```python
from build123d import *

# Parameters (mm, degrees)
SKETCH1_R      = 2
EXTRUDE1_DEPTH = 12
CHAMFER1_SIZE  = 0.25
CHAMFER2_SIZE  = 0.5
EXTRUDE2_DEPTH = 1.5


with BuildPart() as part:
    # Sketch1 → Extrude1 (new body)
    with BuildSketch(Plane(origin=(0, 0, 0), x_dir=(1, 0, 0), z_dir=(0, 1, 0))):
        with Locations(Location((0, 0, 0), (0, 0, 270))):
            Circle(SKETCH1_R)
    extrude(amount=EXTRUDE1_DEPTH)

    # Chamfer1
    chamfer1_edges = [part.edges().sort_by_distance(p)[0] for p in [
        (0, 12, -2),
    ]]
    chamfer(chamfer1_edges, length=CHAMFER1_SIZE)

    # Chamfer2
    chamfer2_edges = [part.edges().sort_by_distance(p)[0] for p in [
        (0, 0, -2),
    ]]
    chamfer(chamfer2_edges, length=CHAMFER2_SIZE)

    # Sketch2 → Extrude2 (cut)
    with BuildSketch(Plane(origin=(0, 12, 0), x_dir=(1, 0, 0), z_dir=(0, 1, 0))):
        Polygon((-1.154700538, 0), (-0.577350269, -1), (0.577350269, -1), (1.154700538, 0), (0.577350269, 1), (-0.577350269, 1), align=None)
    extrude(amount=-EXTRUDE2_DEPTH, mode=Mode.SUBTRACT)


solid = part.part
```
The model under review builds one solid part; all positions refer to its coordinate system, in mm. A direction names the side the tool comes from. Round coordinates to 2 decimals unless told otherwise and drop trailing zeros. Loops run counter-clockwise (first coordinate to the right, second up) from the corner with the lowest first, then second, coordinate; pieces in that order, holes last. Notation, with made-up numbers: (82.25, -24.5) - (123.25, -24.5) arc R8 ccw to (123.25, -18.5) - close; hole circle Ø1 at (53.5, 32). An arc over 180 degrees is marked (long way). Use a Markdown table: item, result. Add a question column.
Q1. For probe 1 along Y at (x, z) = (0.8, -0.35); probe 2 along Z at (x, y) = (-1.5, 1.5); probe 3 along X at (y, z) = (7, -1.7), list the stretches that pass through material, from the lowest coordinate up.
Q2. Insertion check: pin 1 Ø1.5 at (y, z) = (8.5, -1) entering from -X. The pin has a flat end and moves straight along its axis. Give the tip position at first contact, or say it passes through.
Q3. The part is to be moulded in two halves that separate along Z. For faces 3 (the face through (-2, 6, 0)), 4 (the face through (0, 10.5, 0)), 5 (the face through (0, 0, 0)), say which applies: pulls with the +Z half, pulls with the -Z half, needs draft (parallel to the pull), parting line crosses it, or undercut.
Q4. Machinability: for faces 1 (the face through (0.86, 11.26, 0.51)), 2 (the face through (-1, 12, 1)), which of the approach directions +Z, -Z, +X, -X, +Y, -Y give a long, thin tool a straight path to every point of the face, cutting with its end or side? Answer none if there is none.
Q5. Add section A-A (y = 11.25). State the section outline as (x, z) points.
Q6. Add section B-B (x = 0). State the section outline as (y, z) points, plus the area to 3 significant figures.
Worked answers:
| question | item | result |
|---|---|---|
| 1 | probe 1 | 0 to 10.5 |
| 1 | probe 2 | -1.32 to 1.32 |
| 1 | probe 3 | -1.05 to 1.05 |
| 2 | pin 1 | x = -1.98 |
| 3 | face 3 | parting line crosses it |
| 3 | face 4 | undercut |
| 3 | face 5 | needs draft |
| 4 | face 1 | +Y |
| 4 | face 2 | +Z, -Z, +X, -X, +Y |
| 5 | outline | circle Ø4 at (0, 0); hole (-1.15, 0) - (-0.58, -1) - (0.58, -1) - (1.15, 0) - (0.58, 1) - (-0.58, 1) - close |
| 6 | outline | (0, -1.5) - (0.5, -2) - (11.75, -2) - (12, -1.75) - (12, -1) - (10.5, -1) - (10.5, 1) - (12, 1) - (12, 1.75) - (11.75, 2) - (0.5, 2) - (0, 1.5) - close |
| 6 | area | 44.7 mm² |
